Can you work these out from the model? Positions are in its coordinate system, mm. A direction names the side the tool comes from. Coordinates: 2 decimals unless noted, no trailing zeros. Loops run counter-clockwise (first coordinate to the right, second up) from the corner with the lowest first, then second, coordinate; pieces in that order, holes last. Notation, with made-up numbers: M 79.5,16 L 128.5,16 A30 cw 128.5,50 Z; hole C 64,58.5 d6. An arc over 180 degrees is marked long. Answer as a JSON object with one key per item and string values. Group by question number.
Item 1: If I drill on line 1 (Z direction, x = 0, y = 8.5); line 2 (X direction, y = 12.25, z = -8); line 3 (X direction, y = 2.75, z = 6.5), over which ranges is the centre line in solid material (lowest first)?
Item 2: Which directions (+Z, -Z, +X, -X, +Y, -Y) give clear straight access to the entire face, cutting with the end or side of a thin tool? Please do faces 4 (the flat face through (-4, 6, -22.177)), 5 (the flat face through (15, 6, 3.223)), 6 (the flat face through (2, 5.08, -15)), 7 (the flat face through (-1.268, 6.3, 6.8)).
Item 3: I'm going to push flat-ended pins straight in: pin 1 Ø15 at (x, z) = (5.08, -9.48) entering from -Y; pin 2 Ø1.5 at (x, y) = (12, 8.5) entering from -Z; pin 3 Ø3 at (x, y) = (-6, 5) entering from +Z; pin 4 Ø1.9 at (x, y) = (-4, 6.5) entering from -Z. Where does each tip first touch, or does it pass through?
Item 4: Suppose I cut it at A-A (y = 5.75). Write out the boundary of the cut face in (x, z) (3 decimals), then the cut area to 3 significant figures.
Item 5: Suppose I cut it at B-B (x = 8). Count the separate pieces of the cut face and the enclosed holes in it, then the cut area to 3 significant figures.
Item 6: We'd pull the mould along Z, two halves only. Please class faces 1 (the cylindrical face through (5.171, 1.909, 14.113)), 2 (the cylindrical face through (5.171, 5.389, -30.844)), 3 (the flat face through (11.432, 6.3, 6.8)): +Z half, -Z half, draft (parallel to the pull), parting line (faces both ways), or undercut.
Item 7: Suppose I cut it at C-C (y = 2). Write out the boundary of the cut face in (x, z) (3 decimals).
Item 8: Suppose I cut it at D-D (z = 1). Write out the boundary of the cut face in (x, y).
Autodesk Inventor part; units mm, degrees
ref_plane "YZ Plane" through (0, 0, 0) normal (1, 0, 0) x (0, 1, 0)
ref_plane "XZ Plane" through (0, 0, 0) normal (0, 1, 0) x (-1, 0, 0)
ref_plane "XY Plane" through (0, 0, 0) normal (0, 0, 1) x (1, 0, 0)
sketch "Sketch1" plane through (0, 0, 0) normal (0, 1, 0) x (-1, 0, 0)
  line L0 (7.6182, 15.9234) -> (-17.7818, 15.9234)
  line L1 (-17.7818, 15.9234) -> (-17.7818, -34.8766)
  line L2 (-17.7818, -34.8766) -> (7.6182, -34.8766)
  line L3 (7.6182, -34.8766) -> (7.6182, 15.9234)
  line L4 (7.6182, 15.9234) -> (1.2682, 15.9234)
  line L5 (1.2682, 15.9234) -> (1.2682, 3.2234)
  line L6 (1.2682, 3.2234) -> (7.6182, 3.2234)
  line L7 (7.6182, 3.2234) -> (7.6182, 15.9234)
  line L8 (-17.7818, 15.9234) -> (-11.4318, 15.9234)
  line L9 (-11.4318, 15.9234) -> (-11.4318, 3.2234)
  line L10 (-11.4318, 3.2234) -> (-17.7818, 3.2234)
  line L11 (-17.7818, 3.2234) -> (-17.7818, 15.9234)
  line L12 (-17.7818, -34.8766) -> (-11.4318, -34.8766)
  line L13 (-11.4318, -34.8766) -> (-11.4318, -22.1766)
  line L14 (-11.4318, -22.1766) -> (-17.7818, -22.1766)
  line L15 (-17.7818, -22.1766) -> (-17.7818, -34.8766)
  line L16 (7.6182, -34.8766) -> (1.2682, -34.8766)
  line L17 (1.2682, -34.8766) -> (1.2682, -22.1766)
  line L18 (1.2682, -22.1766) -> (7.6182, -22.1766)
  line L19 (7.6182, -22.1766) -> (7.6182, -34.8766)
  circle A0 centre (-5.0818, -9.4766) radius 5.715
  point P0 (0, 0)
  dimension "d0" = 25.4
  dimension "d1" = 50.8
  dimension "d2" = 6.35
  dimension "d3" = 12.7
  dimension "d4" = 6.35
  dimension "d5" = 12.7
  dimension "d6" = 6.35
  dimension "d7" = 12.7
  dimension "d8" = 11.43
extrude "Extrusion1" add sketch "Sketch1" along normal blind 12.7 contours L5 L6 L3 L18 L17 L2 L13 L14 L1 L10 L9 L0
sketch "Sketch2" plane through (11.4318, 0, 3.2234) normal (1, 0, 0) x (0, 0, -1)
  line L0 (-12.7, 0) -> (-12.7, 12.7)
  line L1 (-12.7, 12.7) -> (0, 12.7)
  line L2 (38.1, 12.7) -> (38.1, 0)
  circle A0 centre (-6.35, 6.35) radius 2.5083
  circle A1 centre (31.75, 6.35) radius 2.5082
  point P0 (3.2234, 0)
  dimension "d11" = 6.35
  dimension "d12" = 6.35
  dimension "d13" = 6.35
  dimension "d14" = 5.0165
  dimension "d15" = 5.0165
extrude "Extrusion2" cut sketch "Sketch2" against normal through all
sketch "Sketch3" plane through (0, 12.7, 0) normal (0, 1, 0) x (1, 0, 0)
  circle A0 centre (5.0818, 9.4766) radius 5.715
  circle A1 centre (5.0818, 9.4766) radius 11.176
  point P0 (0, 0)
  dimension "d18" = 22.352
extrude "Extrusion3" cut sketch "Sketch3" against normal blind 7.62
fillet "Fillet1" radius 6.35 4 edges at (5.0818, 12.7, 15.9234) (5.0818, 0, 15.9234) (5.0818, 0, -34.8766) (5.0818, 12.7, -34.8766)
properties part number "top_anchor_v3"
From the geometry:
{
 "1": {"line 1": "-34.5 to -29.82, -27.23 to -19.43, 0.48 to 8.28, 10.87 to 15.55", "line 2": "-7.62 to -6, 16.16 to 17.78", "line 3": "-1.27 to 11.43"},
 "2": {"face 4": "-Z, -X, +Y, -Y", "face 5": "+Z, +X, +Y, -Y", "face 6": "+Y", "face 7": "+Z, -X, +Y, -Y"},
 "3": {"pin 1": "y = 0", "pin 2": "z = -34.66", "pin 3": "z = 3.22", "pin 4": "z = -22.18"},
 "4": {"outline": "M -7.618,-22.177 L -1.268,-22.177 L -1.268,-26.091 L 11.432,-26.091 L 11.432,-22.177 L 17.782,-22.177 L 17.782,3.223 L 11.432,3.223 L 11.432,7.138 L -1.268,7.138 L -1.268,3.223 L -7.618,3.223 Z; M -1.268,-34.848 L 11.432,-34.848 L 11.432,-30.962 L -1.268,-30.962 Z; M -1.268,12.009 L 11.432,12.009 L 11.432,15.895 L -1.268,15.895 Z; hole C 5.082,-9.477 d22.352", "area": "451 mm2"},
 "5": {"separate pieces": "2", "enclosed holes": "2", "area": "357 mm2"},
 "6": {"face 1": "+Z half", "face 2": "undercut", "face 3": "draft"},
 "7": {"outline": "M -7.618,-22.177 L -1.268,-22.177 L -1.268,-33.153 L 11.432,-33.153 L 11.432,-22.177 L 17.782,-22.177 L 17.782,3.223 L 11.432,3.223 L 11.432,14.199 L -1.268,14.199 L -1.268,3.223 L -7.618,3.223 Z; hole C 5.082,-9.477 d11.43"},
 "8": {"outline": "M -7.62,0 L 17.78,0 L 17.78,12.7 L 8.97,12.7 L 8.97,5.08 L 1.19,5.08 L 1.19,12.7 L -7.62,12.7 Z"}
}
